from build123d import *

# Parameters (mm, degrees)
PAD_DEPTH       = 3
SKETCH001_W     = 59
SKETCH001_H     = 49
POCKET_DEPTH    = 2
SKETCH002_W     = 12
SKETCH002_H     = 14
PAD001_DEPTH    = 24
SKETCH003_R     = 2
SKETCH003_R_2   = 1.5
SKETCH003_W     = 5
SKETCH003_H     = 4
POCKET001_DEPTH = 3.001
SKETCH004_R     = 10
POCKET002_DEPTH = 2
SKETCH005_R     = 2
POCKET003_DEPTH = 18


with BuildPart() as part:
    # Sketch → Pad (new body)
    with BuildSketch(Plane(origin=(0, 150, 0), x_dir=(1, 0, 0), z_dir=(0, 0, 1))):
        Polygon((-26, 47), (-26, -47), (128, -47), (148, -37), (148, 37), (128, 47), align=None)
    extrude(amount=PAD_DEPTH)

    # Sketch001 → Pocket (cut)
    with BuildSketch(Plane(origin=(0, 150, 3), x_dir=(1, 0, 0), z_dir=(0, 0, 1))):
        with Locations((29.5, 0)):
            Rectangle(SKETCH001_W, SKETCH001_H)
    extrude(amount=-POCKET_DEPTH, mode=Mode.SUBTRACT)

    # Sketch002 → Pad001 (new body)
    with BuildSketch(Plane(origin=(0, 150, 3), x_dir=(1, 0, 0), z_dir=(0, 0, 1))):
        with Locations((65, 40)):
            Rectangle(SKETCH002_W, SKETCH002_H)
        with Locations((65, -40)):
            Rectangle(SKETCH002_W, SKETCH002_H)
        Polygon((103, 29), (125, 29), (125, 47), (113, 47), (113, 33), (103, 33), align=None)
        Polygon((103, -29), (125, -29), (125, -47), (113, -47), (113, -33), (103, -33), align=None)
    extrude(amount=PAD001_DEPTH)

    # Sketch003 → Pocket001 (cut, through all)
    with BuildSketch(Plane(origin=(0, 150, 3), x_dir=(1, 0, 0), z_dir=(0, 0, 1))):
        with Locations((-12, 0)):
            Circle(SKETCH003_R)
        with Locations((142, 5)):
            Circle(SKETCH003_R_2)
        with Locations((142, -5)):
            Circle(SKETCH003_R_2)
        with Locations((93.5, 31)):
            Rectangle(SKETCH003_W, SKETCH003_H)
        with Locations((93.5, -31)):
            Rectangle(SKETCH003_W, SKETCH003_H)
    extrude(amount=-POCKET001_DEPTH, mode=Mode.SUBTRACT)

    # Sketch004 → Pocket002 (cut)
    with BuildSketch(Plane(origin=(0, 150, 0), x_dir=(1, 0, 0), z_dir=(0, 0, -1))):
        with Locations((-12, 0)):
            Circle(SKETCH004_R)
    extrude(amount=-POCKET002_DEPTH, mode=Mode.SUBTRACT)

    # Sketch005 → Pocket003 (cut)
    with BuildSketch(Plane(origin=(0, 150, 27), x_dir=(1, 0, 0), z_dir=(0, 0, 1))):
        with Locations((119, 40)):
            Circle(SKETCH005_R)
        with Locations((65, 40)):
            Circle(SKETCH005_R)
        with Locations((119, -40)):
            Circle(SKETCH005_R)
        with Locations((65, -40)):
            Circle(SKETCH005_R)
    extrude(amount=-POCKET003_DEPTH, mode=Mode.SUBTRACT)


solid = part.part
Here's how the part is built. I have some questions about the finished solid (model axes, mm). A direction names the side the tool comes from. Round coordinates to 2 decimals unless told otherwise and drop trailing zeros. Loops run counter-clockwise (first coordinate to the right, second up) from the corner with the lowest first, then second, coordinate; pieces in that order, holes last.
1. If I drill on line 1 along Y through (x, z) = (65, 17.25); line 2 along Y through (x, z) = (119, 16); line 3 along X through (y, z) = (190, 23.5), over which ranges is the centre line in solid material (lowest first)?
Answer list:
line 1: y = 103 to 108, 112 to 117, 183 to 188, 192 to 197
line 2: y = 103 to 108, 112 to 121, 179 to 188, 192 to 197
line 3: x = 59 to 63, 67 to 71, 113 to 117, 121 to 125
2. We'd pull the mould along Y, two halves only. Please class faces 1 (the face through (138, 108, 1)), 2 (the face through (-14.17, 159.76, 0.99)), 3 (the face through (148, 149, 1)): +Y half, -Y half, draft (parallel to the pull), parting line (faces both ways), or undercut.
Answer list:
face 1: -Y half
face 2: undercut
face 3: draft
3. If we section it at A-A on z = 19.5: Write out the boundary of the cut face in (x, y).
Answer list:
outline: (59, 103) - (71, 103) - (71, 117) - (59, 117) - close; (59, 183) - (71, 183) - (71, 197) - (59, 197) - close; (103, 117) - (113, 117) - (113, 103) - (125, 103) - (125, 121) - (103, 121) - close; (103, 179) - (125, 179) - (125, 197) - (113, 197) - (113, 183) - (103, 183) - close; hole circle Ø4 at (65, 110); hole circle Ø4 at (65, 190); hole circle Ø4 at (119, 110); hole circle Ø4 at (119, 190)
4. Which directions (+Z, -Z, +X, -X, +Y, -Y) give clear straight access to the entire face, cutting with the end or side of a thin tool? Please do faces 4 (the face through (96, 181, 2)), 5 (the face through (125, 112, 15)), 6 (the face through (117.4, 188.8, 18.1)).
Answer list:
face 4: +Z, -Z
face 5: +Z, +X, +Y, -Y
face 6: +Z
5. If we section it at B-B on x = -12: Write out the boundary of the cut face in (y, z), plus the area to 3 significant figures.
Answer list:
outline: (103, 0) - (140, 0) - (140, 2) - (148, 2) - (148, 3) - (103, 3) - close; (152, 2) - (160, 2) - (160, 0) - (197, 0) - (197, 3) - (152, 3) - close
area: 238 mm2
6. If we section it at C-C on y = 150: Write out the boundary of the cut face in (x, z).
Answer list:
outline: (-26, 0) - (-22, 0) - (-22, 2) - (-14, 2) - (-14, 3) - (-26, 3) - close; (-10, 2) - (-2, 2) - (-2, 0) - (148, 0) - (148, 3) - (59, 3) - (59, 1) - (0, 1) - (0, 3) - (-10, 3) - close
7. For P1, Ø4.5, axis at y = 119.5, z = 19.5, coming from the -X side; P2, Ø5, axis at x = -12, y = 150, coming from the -Z side; P3, Ø4, axis at x = 142, y = 155, coming from the +Z side, each with a flat end and sliding along its axis, tell me the tip position at first contact or that it passes through.
Answer list:
P1: stops at x = 103
P2: stops at z = 2
P3: stops at z = 3
8. If we section it at D-D on y = 110: Write out the boundary of the cut face in (x, z).
Answer list:
outline: (-26, 0) - (142, 0) - (142, 3) - (125, 3) - (125, 27) - (121, 27) - (121, 9) - (117, 9) - (117, 27) - (113, 27) - (113, 3) - (71, 3) - (71, 27) - (67, 27) - (67, 9) - (63, 9) - (63, 27) - (59, 27) - (59, 3) - (-26, 3) - close
